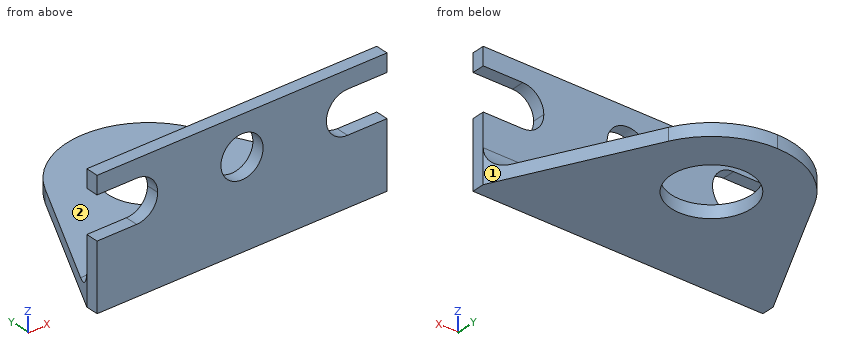
from build123d import *

# Parameters (mm, degrees)
SKETCH1_R               = 4.826
EXTRUDE1_DEPTH          = 1.524
SKETCH2_W               = 34.925
SKETCH2_H               = 1.524
EXTRUDE2_DEPTH          = 15.24
SKETCH3_R               = 2.54
CUT_EXTRUDE1_DEPTH      = 33.199509472
CUT_EXTRUDE2_DEPTH      = 33.199509472
CUT_EXTRUDE2_DEPTH_BACK = 33.199509472
FILLET1_R               = 2.54


with BuildPart() as part:
    # Sketch1 → Extrude1 (new body)
    with BuildSketch(Plane.XY):
        with BuildLine():
            Line((-17.4625, 0), (17.4625, 0))
            Line((17.4625, 0), (17.4625, 1.524))
            Line((17.4625, 1.524), (8.825639974, 18.468545882))
            ThreePointArc((8.825639974, 18.468545882), (5.175241081, 22.416639317), (0, 23.876))
            ThreePointArc((0, 23.876), (-5.175241081, 22.416639317), (-8.825639974, 18.468545882))
            Line((-8.825639974, 18.468545882), (-17.4625, 1.524))
            Line((-17.4625, 1.524), (-17.4625, 0))
        make_face()
        with Locations(Location((0, 13.97, 0), (0, 0, 180))):
            Circle(SKETCH1_R, mode=Mode.SUBTRACT)
    extrude(amount=EXTRUDE1_DEPTH)

    # Sketch2 → Extrude2 (add)
    with BuildSketch(Plane(origin=(0, 0, 0), x_dir=(-1, 0, 0), z_dir=(0, 0, -1))):
        with Locations((0, 0.762)):
            Rectangle(SKETCH2_W, SKETCH2_H)
    extrude(amount=-EXTRUDE2_DEPTH)

    # Sketch3 → Cut-Extrude1 (cut, through all)
    with BuildSketch(Plane(origin=(0, 1.524, 0), x_dir=(-1, 0, 0), z_dir=(0, 1, 0))):
        with Locations(Location((0, 10.541, 0), (0, 0, 90))):
            Circle(SKETCH3_R)
    extrude(amount=-CUT_EXTRUDE1_DEPTH, mode=Mode.SUBTRACT)

    # Sketch4 → Cut-Extrude2 (cut, two sides)
    with BuildSketch(Plane(origin=(0, 1.524, 0), x_dir=(-1, 0, 0), z_dir=(0, 1, 0))) as cut_extrude2_sk:
        with BuildLine():
            Line((12.7, 8.001), (17.4625, 8.001))
            Line((17.4625, 8.001), (17.4625, 13.081))
            Line((17.4625, 13.081), (12.7, 13.081))
            ThreePointArc((12.7, 13.081), (10.903948776, 12.337051224), (10.16, 10.541))
            ThreePointArc((10.16, 10.541), (10.903948776, 8.744948776), (12.7, 8.001))
        make_face()
    cut_extrude2 = extrude(amount=CUT_EXTRUDE2_DEPTH, mode=Mode.SUBTRACT)
    cut_extrude2 = cut_extrude2 + extrude(cut_extrude2_sk.sketch, amount=-CUT_EXTRUDE2_DEPTH_BACK, mode=Mode.SUBTRACT)

    # Mirror1: Cut-Extrude2 across plane
    add(cut_extrude2.mirror(Plane(origin=(0, 0, 0), x_dir=(0, 0, 1), z_dir=(1, 0, 0))), mode=Mode.SUBTRACT)

    # Fillet1
    fillet1_edges = [part.edges().sort_by_distance(p)[0] for p in [
        (0, 1.524, 1.524),
    ]]
    fillet(fillet1_edges, radius=FILLET1_R)


solid = part.part
Verification items for the finished model (mm, model axes). Face numbers are marked on the shaded views. A direction names the side the tool comes from. Give positions to 0.01 mm unless a question says otherwise; leave off trailing zeros. Write each loop counter-clockwise with the first axis right and the second up, starting at its lowest first coordinate (ties: lowest second). Pieces come first, ordered by that corner, then holes.
(1) Cross-section at B-B (y = 9.75). Enter the section's corners in (x, z).
(2) Cross-section at D-D (z = 3). Enter the section's corners in (x, y), plus the area to 3 significant figures.
(3) Gauge pin test, flat ends, axial feed: pin 1 (8 mm diameter, centred on y = 6, z = 7.5, fed in from +X); pin 2 (8 mm diameter, centred on x = 12, z = 13.5, fed in from +Y); pin 3 (1.5 mm diameter, centred on x = 9.5, y = 8, fed in from +Z). Record the tip position at first contact, or that the pin passes through.
(4) Access from +Z, -Z, +X, -X, +Y, -Y to the whole of each face (thin tool, end or side, straight path). Record for the marked faces 1 and 2.
(5) Cross-section at A-A (z = 9.5). Enter the section's corners in (x, y).
(6) Material ranges on line 1 (Y direction, x = 14.5, z = 5.75); line 2 (X direction, y = 13.97, z = 0.6), recorded low to high.
(7) Cross-section at C-C (x = -3). Enter the section's corners in (y, z), plus the area to 3 significant figures.
Worked out:
1. outline: (-13.27, 0) - (-2.34, 0) - (-2.34, 1.52) - (-13.27, 1.52) - close; (2.34, 0) - (13.27, 0) - (13.27, 1.52) - (2.34, 1.52) - close
2. outline: (-17.46, 0) - (17.46, 0) - (17.46, 1.52) - (17.34, 1.76) - (-17.34, 1.76) - (-17.46, 1.52) - close
2. area: 61.4 mm2
3. pin 1: passes through
3. pin 2: stops at y = 1.52
3. pin 3: stops at z = 1.52
4. face 1: +Z, -Z, +X, +Y
4. face 2: +Z, +X, -X, +Y
5. outline: (-10.38, 0) - (-2.32, 0) - (-2.32, 1.52) - (-10.38, 1.52) - close; (2.32, 0) - (10.38, 0) - (10.38, 1.52) - (2.32, 1.52) - close
6. line 1: y = 0 to 1.52
6. line 2: x = -11.12 to -4.83, 4.83 to 11.12
7. outline: (0, 0) - (10.19, 0) - (10.19, 1.52) - (4.06, 1.52) arc R2.54 cw to (1.52, 4.06) - (1.52, 15.24) - (0, 15.24) - close; (17.75, 0) - (23.41, 0) - (23.41, 1.52) - (17.75, 1.52) - close
7. area: 46.4 mm2
